```python
from build123d import *

# Parameters (mm, degrees)
BASE_EXTRUDE_DEPTH           = 203.2
TAP_DRILL_FOR_M10X1_0_TAP2_D = 9
LPATTERN1_COUNT              = 4
LPATTERN1_PITCH              = 50.8


with BuildPart() as part:
    # Sketch1 → Base-Extrude (new body)
    with BuildSketch(Plane.XY):
        with BuildLine():
            Line((-51.848409542, -29.029859377), (-51.848409542, -32.936966461))
            Line((-51.848409542, -32.936966461), (-66.799126207, -32.936966461))
            Line((-66.799126207, -32.936966461), (-68.5063829, -31.355514763))
            Line((-68.5063829, -31.355514763), (-68.5063829, 11.513033539))
            Line((-68.5063829, 11.513033539), (-3.9903829, 11.513033539))
            Line((-3.9903829, 11.513033539), (-3.9903829, -31.355514763))
            Line((-3.9903829, -31.355514763), (-5.697639593, -32.936966461))
            Line((-5.697639593, -32.936966461), (-20.648356257, -32.936966461))
            Line((-20.648356257, -32.936966461), (-20.648356257, -29.029859377))
            ThreePointArc((-20.648356257, -29.029859377), (-17.301518569, -17.177491216), (-27.3583829, -10.068382033))
            Line((-27.3583829, -10.068382033), (-45.1383829, -10.068382033))
            ThreePointArc((-45.1383829, -10.068382033), (-55.19524723, -17.177491216), (-51.848409542, -29.029859377))
        make_face()
    extrude(amount=BASE_EXTRUDE_DEPTH)

    # Tap Drill for M10x1.0 Tap2 (through all)
    with Locations(Plane(origin=(0, 11.513033539, 0), x_dir=(-1, 0, 0), z_dir=(0, 1, 0))):
        with Locations((36.2483829, 177.8)):
            tap_drill_for_m10x1_0_tap2 = Hole(TAP_DRILL_FOR_M10X1_0_TAP2_D / 2)

    # LPattern1: Tap Drill for M10x1.0 Tap2 ×4
    with Locations(*[(0, 0, -i * LPATTERN1_PITCH) for i in range(1, LPATTERN1_COUNT)]):
        add(tap_drill_for_m10x1_0_tap2, mode=Mode.SUBTRACT)


solid = part.part
```
Here's how the part is built. I have some questions about the finished solid (model axes, mm). A direction names the side the tool comes from. Round coordinates to 2 decimals unless told otherwise and drop trailing zeros. Loops run counter-clockwise (first coordinate to the right, second up) from the corner with the lowest first, then second, coordinate; pieces in that order, holes last.
1. Suppose I cut it at D-D, the plane z = 180.5. Please give me the cut outline in (x, y), and give its area (3 significant figures).
Answers:
outline: (-68.51, -31.36) - (-66.8, -32.94) - (-51.85, -32.94) - (-51.85, -29.03) arc R10.67 cw to (-45.14, -10.07) - (-39.85, -10.07) - (-39.85, 11.51) - (-68.51, 11.51) - close; (-32.65, -10.07) - (-27.36, -10.07) arc R10.67 cw to (-20.65, -29.03) - (-20.65, -32.94) - (-5.7, -32.94) - (-3.99, -31.36) - (-3.99, 11.51) - (-32.65, 11.51) - close
area: 1,910 mm2
2. Suppose I cut it at B-B, the plane y = 5. Please give me the cut outline in (x, z), and give its area (3 significant figures).
Answers:
outline: (-68.51, 0) - (-3.99, 0) - (-3.99, 203.2) - (-68.51, 203.2) - close; hole circle Ø9 at (-36.25, 25.4); hole circle Ø9 at (-36.25, 76.2); hole circle Ø9 at (-36.25, 127); hole circle Ø9 at (-36.25, 177.8)
area: 12,900 mm2
3. Will these pins go through, and if not, where does the flat tip stop? pin 1 (1 mm diameter, centred on x = -23.5, z = 112.5, fed in from -Y); pin 2 (19.5 mm diameter, centred on x = -35, z = 95.5, fed in from -Y); pin 3 (10.5 mm diameter, centred on x = -36.25, z = 76.2, fed in from -Y).
Answers:
pin 1: stops at y = -11
pin 2: stops at y = -10.28
pin 3: stops at y = -10.07
4. Thinking about a two-plate mould opening in X: for faces 4 (the face through (-13, -32.937, 100)), 5 (the face through (-3.99, -10, 100)), 6 (the face through (-33.829, 0.571, 79.994)), 7 (the face through (-68.506, -10, 100)), which applies, released by +X, released by -X, zero draft, split by the parting line, or undercut?
Answers:
face 4: zero draft
face 5: released by +X
face 6: undercut
face 7: released by -X
5. Suppose I cut it at A-A, the plane z = 25.4. Please give me the cut outline in (x, y).
Answers:
outline: (-68.51, -31.36) - (-66.8, -32.94) - (-51.85, -32.94) - (-51.85, -29.03) arc R10.67 cw to (-45.14, -10.07) - (-40.75, -10.07) - (-40.75, 11.51) - (-68.51, 11.51) - close; (-31.75, -10.07) - (-27.36, -10.07) arc R10.67 cw to (-20.65, -29.03) - (-20.65, -32.94) - (-5.7, -32.94) - (-3.99, -31.36) - (-3.99, 11.51) - (-31.75, 11.51) - close
6. Suppose I cut it at C-C, the plane y = -16. Please give me the cut outline in (x, z), and give its area (3 significant figures).
Answers:
outline: (-68.51, 0) - (-54.7, 0) - (-54.7, 203.2) - (-68.51, 203.2) - close; (-17.8, 0) - (-3.99, 0) - (-3.99, 203.2) - (-17.8, 203.2) - close
area: 5,610 mm2
7. If I drill on probe 1 along X at (y, z) = (2, 76); probe 2 along Z at (x, y) = (-35, -2.5); probe 3 along X at (y, z) = (-20, 141), over which ranges is the centre line in solid material (lowest first)?
Answers:
probe 1: x = -68.51 to -40.74, -31.75 to -3.99
probe 2: z = 0 to 21.08, 29.72 to 71.88, 80.52 to 122.68, 131.32 to 173.48, 182.12 to 203.2
probe 3: x = -68.51 to -55.78, -16.72 to -3.99
8. For faces 1 (the face through (-34.17, 0.57, 123.01)), 2 (the face through (-55.13, -17, 100.18)), 3 (the face through (-36, -10.068, 100)), which set-ups out of +Z, -Z, +X, -X, +Y, -Y let a thin tool reach every point of the face, with its end or its side?
Answers:
face 1: +Y, -Y
face 2: +Z, -Z
face 3: +Z, -Z, -Y
